For this review, take the finished solid that the model builds, in its own axes (mm). Give positions to 0.01 mm unless a question says otherwise; leave off trailing zeros. Write each loop counter-clockwise with the first axis right and the second up, starting at its lowest first coordinate (ties: lowest second). Pieces come first, ordered by that corner, then holes.
Q1. We need section C-C (x = 20). Write out the cut boundary in (y, z).
Q2. Mouldability with a two-part tool opening along X and no side actions: class faces 1 (the cylindrical face through (-20.358, 20.727, 29.812)), 2 (the flat face through (25, -5.8, 31.4)), 3 (the cylindrical face through (19.404, -24.685, 28.171)), 4 (the flat face through (0, -27, 25)) as released by +X, released by -X, zero draft, split by the parting line, or undercut.
Q3. We need section D-D (z = 20.5). Write out the cut boundary in (x, y), then the cut area to 3 significant figures.
Q4. For line 1 (X direction, y = 18, z = 31); line 2 (Y direction, x = 20, z = 29.25); line 3 (Y direction, x = -20, z = 27.75), list the stretches that pass through material, from the lowest coordinate up.
Q5. Insertion check: P1, Ø5, axis at x = -20, y = 18, coming from the +Z side; P2, Ø2, axis at x = -10, y = -10.5, coming from the -Z side; P3, Ø10, axis at x = -20, y = -14.5, coming from the -Z side; P4, Ø7, axis at x = -20, y = -22, coming from the +Z side. Each pin has a flat end and moves straight along its axis. Give the tip position at first contact, or say it passes through.
Q6. We need section A-A (z = 28.5). Write out the cut boundary in (x, y).
Q7. We need section B-B (y = -22). Write out the cut boundary in (x, z), then the cut area to 3 significant figures.
```python
from build123d import *

# Parameters (mm, degrees)
SKETCH1_W               = 50
SKETCH1_H               = 50
SKETCH1_R               = 2.75
BOSS_EXTRUDE1_DEPTH     = 33.6
CUT_EXTRUDE1_DEPTH      = 50.829308645
CUT_EXTRUDE1_DEPTH_BACK = 50.829308645
SKETCH2_R               = 31.75


with BuildPart() as part:
    # Sketch1 → Boss-Extrude1 (new body)
    with BuildSketch(Plane.XY):
        with Locations((0, -2)):
            Rectangle(SKETCH1_W, SKETCH1_H)
        with Locations((-20, 18)):
            Circle(SKETCH1_R, mode=Mode.SUBTRACT)
        with Locations((20, 18)):
            Circle(SKETCH1_R, mode=Mode.SUBTRACT)
        with Locations((20, -22)):
            Circle(SKETCH1_R, mode=Mode.SUBTRACT)
        with Locations((-20, -22)):
            Circle(SKETCH1_R, mode=Mode.SUBTRACT)
    extrude(amount=BOSS_EXTRUDE1_DEPTH)

    # Sketch2 → Cut-Extrude1 (cut, two sides: drawn at the far end of the back side and taken through both)
    with BuildSketch(Plane(origin=(0, 0, 0), x_dir=(0, 0, -1), z_dir=(1, 0, 0)).offset(-CUT_EXTRUDE1_DEPTH_BACK)):
        Circle(SKETCH2_R)
    extrude(amount=CUT_EXTRUDE1_DEPTH + CUT_EXTRUDE1_DEPTH_BACK, mode=Mode.SUBTRACT)


solid = part.part
```
Computed:
1. outline: (-27, 16.71) arc R31.75 cw to (-24.75, 19.89) - (-24.75, 33.6) - (-27, 33.6) - close; (-19.25, 25.25) arc R31.75 cw to (15.25, 27.85) - (15.25, 33.6) - (-19.25, 33.6) - close; (20.75, 24.03) arc R31.75 cw to (23, 21.89) - (23, 33.6) - (20.75, 33.6) - close
2. face 1: undercut
2. face 2: released by +X
2. face 3: undercut
2. face 4: zero draft
3. outline: (-25, -27) - (25, -27) - (25, -24.24) - (21.59, -24.24) arc R2.75 cw to (18.41, -24.24) - (-18.41, -24.24) arc R2.75 cw to (-21.59, -24.24) - (-25, -24.24) - close
3. area: 136 mm2
4. line 1: x = -25 to -22.75, -17.25 to 17.25, 22.75 to 25
4. line 2: y = -27 to -24.75, -19.25 to -12.35, 12.35 to 15.25, 20.75 to 23
4. line 3: y = -27 to -24.75, -19.25 to -15.43, 20.75 to 23
5. P1: passes through
5. P2: stops at z = 29.59
5. P3: stops at z = 25.12
5. P4: stops at z = 33.6
6. outline: (-25, -27) - (25, -27) - (25, -13.99) - (-25, -13.99) - close; (-25, 13.99) - (25, 13.99) - (25, 23) - (-25, 23) - close; hole circle Ø5.5 at (-20, -22); hole circle Ø5.5 at (-20, 18); hole circle Ø5.5 at (20, -22); hole circle Ø5.5 at (20, 18)
7. outline: (-25, 22.89) - (-22.75, 22.89) - (-22.75, 33.6) - (-25, 33.6) - close; (-17.25, 22.89) - (17.25, 22.89) - (17.25, 33.6) - (-17.25, 33.6) - close; (22.75, 22.89) - (25, 22.89) - (25, 33.6) - (22.75, 33.6) - close
7. area: 418 mm2
